```python
from build123d import *

# Parameters (mm, degrees)
SKETCH_R           = 6
PAD_DEPTH          = 4
SKETCH001_R        = 12.5
PAD001_DEPTH       = 3
SKETCH002_R        = 4
POCKET_DEPTH       = 3
POLARPATTERN_COUNT = 5
FILLET_R           = 2
SKETCH003_R        = 2.31
POCKET001_DEPTH    = 3
POCKET001_FACE25_R = 6
POCKET002_DEPTH    = 1
POCKET002_FACE26_R = 2.31
POCKET003_DEPTH    = 1.5
POCKET003_FACE26_R = 2.31
POCKET004_DEPTH    = 1.501
SKETCH005_R        = 6
SKETCH005_R_2      = 2.31
PAD002_DEPTH       = 3
PAD002_FACE38_R    = 2.31
PAD003_DEPTH       = 3
SKETCH006_R        = 4.075
POCKET005_DEPTH    = 6.001


with BuildPart() as part:
    # Sketch → Pad (new body)
    with BuildSketch(Plane.XY):
        Circle(SKETCH_R)
        Polygon((-2.286307, -3.96), (2.286307, -3.96), (4.572614, 0), (2.286307, 3.96), (-2.286307, 3.96), (-4.572614, 0), align=None, mode=Mode.SUBTRACT)
    extrude(amount=PAD_DEPTH)

    # Sketch001 (on Face9 of Pad) → Pad001 (join)
    with BuildSketch(Plane.XY.offset(4)):
        Circle(SKETCH001_R)
    extrude(amount=PAD001_DEPTH)

    # Sketch002 (on Face3 of Pad001) → Pocket (cut)
    with BuildSketch(Plane.XY.offset(7)):
        with Locations((0, 12.5)):
            Circle(SKETCH002_R)
    pocket = extrude(amount=-POCKET_DEPTH, mode=Mode.SUBTRACT)

    # PolarPattern: Pocket ×5 about axis
    polarpattern_axis = Axis((0, 0, 0), (0, 0, 1))
    for i in range(1, POLARPATTERN_COUNT):
        add(pocket.rotate(polarpattern_axis, i * 360 / POLARPATTERN_COUNT), mode=Mode.SUBTRACT)

    # Fillet
    fillet_edges = [part.edges().sort_by_distance(p)[0] for p in [
        (-12.499674, -0.090275, 5.5),
        (-10.059387, 7.420158, 5.5),
        (-3.948468, 11.86, 5.5),
        (3.948468, 11.86, 5.5),
        (-3.776755, -11.915793, 5.5),
        (-10.165511, -7.27409, 5.5),
        (10.165511, -7.27409, 5.5),
        (3.776755, -11.915793, 5.5),
        (10.059387, 7.420158, 5.5),
        (12.499674, -0.090275, 5.5),
    ]]
    fillet(fillet_edges, radius=FILLET_R)

    # Sketch003 (on Face31 of Fillet) → Pocket001 (cut)
    with BuildSketch(Plane(origin=(0, 0, 4), x_dir=(1, 0, 0), z_dir=(0, 0, -1))):
        Circle(SKETCH003_R)
    extrude(amount=-POCKET001_DEPTH, mode=Mode.SUBTRACT)

    # Pocket001 Face25 → Pocket002 (cut)
    with BuildSketch(Plane(origin=(0, 0, 0), x_dir=(0, -1, 0), z_dir=(0, 0, -1))):
        Circle(POCKET001_FACE25_R)
        Polygon((0, 4.572614), (3.96, 2.286307), (3.96, -2.286307), (0, -4.572614), (-3.96, -2.286307), (-3.96, 2.286307), align=None, mode=Mode.SUBTRACT)
    extrude(amount=-POCKET002_DEPTH, mode=Mode.SUBTRACT)

    # Pocket002 Face26 → Pocket003 (cut)
    with BuildSketch(Plane(origin=(0, 0, 4), x_dir=(0, -1, 0), z_dir=(0, 0, -1))):
        Polygon((0, 4.572614), (-3.96, 2.286307), (-3.96, -2.286307), (0, -4.572614), (3.96, -2.286307), (3.96, 2.286307), align=None)
        Circle(POCKET002_FACE26_R, mode=Mode.SUBTRACT)
    extrude(amount=-POCKET003_DEPTH, mode=Mode.SUBTRACT)

    # Pocket003 Face26 → Pocket004 (cut, through all)
    with BuildSketch(Plane(origin=(0, 0, 5.5), x_dir=(0, -1, 0), z_dir=(0, 0, -1))):
        Polygon((0, 4.572614), (-3.96, 2.286307), (-3.96, -2.286307), (0, -4.572614), (3.96, -2.286307), (3.96, 2.286307), align=None)
        Circle(POCKET003_FACE26_R, mode=Mode.SUBTRACT)
    extrude(amount=-POCKET004_DEPTH, mode=Mode.SUBTRACT)

    # Sketch005 (on Face30 of Pocket004) → Pad002 (join)
    with BuildSketch(Plane(origin=(0, 0, 1), x_dir=(1, 0, 0), z_dir=(0, 0, -1))):
        Circle(SKETCH005_R)
        Circle(SKETCH005_R_2, mode=Mode.SUBTRACT)
    extrude(amount=-PAD002_DEPTH)

    # Pad002 Face38 → Pad003 (add)
    with BuildSketch(Plane(origin=(0, 0, 4), x_dir=(0, 1, 0), z_dir=(0, 0, 1))):
        Polygon((0, 4.572614), (-3.96, 2.286307), (-3.96, -2.286307), (0, -4.572614), (3.96, -2.286307), (3.96, 2.286307), align=None)
        Circle(PAD002_FACE38_R, mode=Mode.SUBTRACT)
    extrude(amount=PAD003_DEPTH)

    # Sketch006 (on Face24 of Pad003) → Pocket005 (cut, through all)
    with BuildSketch(Plane.XY.offset(7)):
        Circle(SKETCH006_R)
    extrude(amount=-POCKET005_DEPTH, mode=Mode.SUBTRACT)


solid = part.part
```
Build history of the part. All positions in model axes, mm. A direction names the side the tool comes from. Coordinates: 2 decimals unless noted, no trailing zeros. Order: outer loops, then holes, each group sorted by start corner. A loop starts at its lowest first (then second) coordinate and runs counter-clockwise, first axis right, second up. Notation, with made-up numbers: M 33.25,-27 L 41.25,-27 A26 ccw 41.25,5 Z; hole C 75.25,-16 d11. An arc over 180 degrees is marked long. One line per question, with ' | ' between items. Start each with the question number.
1. Cut at D-D (y = -8.5). Write the cut outline in (x, z).
2. Cut at B-B (y = 3.25). Write the cut outline in (x, z), plus the area to 3 significant figures.
3. Mould opens along Y. For faces 1 (the face through (-11.895, -3.841, 5.479)), 2 (the face through (-3, -3, 7)), 3 (the face through (-8.102, 2.574, 5.521)), 4 (the face through (7.366, 10.099, 5.479)) say: +Y half, -Y half, draft (parallel to the pull), parting line (faces both ways), or undercut.
4. Cut at A-A (x = 0). Write the cut outline in (y, z) (3 decimals), plus the area to 3 significant figures.
5. Cut at C-C (z = 2.75). Write the cut outline in (x, y) (3 decimals).
6. Tool access for faces 5 (the face through (3, -6, 4)), 6 (the face through (11.881, -3.884, 5.479)): list every direction of +Z, -Z, +X, -X, +Y, -Y with a clear straight run to the whole face (end or side of a thin tool).
7. Wall check: line 1 along Y through (x, z) = (0, 5.15) (3 decimals); line 2 along Y through (x, z) = (0, 3.1) (3 decimals); line 3 along X through (y, z) = (-3.75, 2.5). Give the ranges that are in metal, low to high. Write a range as [from, to].
The answers:
1) outline: M -3.69,4 L 3.69,4 L 3.69,7 L -3.69,7 Z
2) outline: M -7.94,4 L -5.04,4 L -5.04,1 L -2.46,1 L -2.46,7 L -7.94,7 Z; M 2.46,1 L 5.04,1 L 5.04,4 L 7.94,4 L 7.94,7 L 2.46,7 Z | area: 48.4 mm2
3) face 1: -Y half | face 2: draft | face 3: undercut | face 4: +Y half
4) outline: M -12.5,4 L -6,4 L -6,1 L -4.075,1 L -4.075,7 L -12.5,7 Z; M 4.075,1 L 6,1 L 6,4 L 8.5,4 L 8.5,7 L 4.075,7 Z | area: 50.1 mm2
5) outline: C 0,0 d12; hole C 0,0 d8.15
6) face 5: -Z | face 6: +Z, -Z, +X, -Y
7) line 1: y = [-12.5, -4.075], [4.075, 8.5] | line 2: y = [-6, -4.075], [4.075, 6] | line 3: x = [-4.68, -1.59], [1.59, 4.68]
